Work out the finished part from the listing and answer in its coordinate system (mm). A direction names the side the tool comes from. Coordinates: 2 decimals unless noted, no trailing zeros. Write each loop counter-clockwise with the first axis right and the second up, starting at its lowest first coordinate (ties: lowest second). Pieces come first, ordered by that corner, then holes. Notation, with made-up numbers: (-30.75, 23) - (11.25, 23) arc R31 cw to (11.25, 53) - close; hole circle Ø6 at (87, 39.25). An arc over 180 degrees is marked (long way). Use a Markdown table: item, result. Add a question column.
(1) The part is cut by section A-A, the plane x = 0. Give the vertices of the cut face in (y, z).
(2) The part is cut by section D-D, the plane y = 7.75. Give the vertices of the cut face in (x, z) (3 decimals).
(3) A tool of negligible diameter and unlimited length cuts with its end or side. For faces 4 (the face through (0, 4, -4.45)), 5 (the face through (-2.961, 8.172, -1.915)), from which of +Z, -Z, +X, -X, +Y, -Y can it reach the whole face along a straight path? Write none if from no direction.
(4) Given pin 1 Ø5.5 at (x, y) = (0, 0) entering from -Z, flat-ended and moving along its own axis, determine where the tip first touches the part or whether it passes through.
(5) For a pull along Y with two mould halves and no side action, classify faces 1 (the face through (0, 10, 0)), 2 (the face through (2.5, 7.8, 0.55)), 3 (the face through (0, 4, 4.45)) as released by +Y, released by -Y, zero draft, split by the parting line, or undercut.
(6) The part is cut by section C-C, the plane z = 1.25. Give the vertices of the cut face in (x, y).
(7) Find the intervals of material crossed by line 1 (Y direction, x = 0, z = -2.8); line 2 (Y direction, x = 2.5, z = -2.3) (3 decimals); line 3 (X direction, y = 8, z = -3.5), in increasing order. Write a range as from..to.
(8) The part is cut by section B-B, the plane z = -3.25. Give the vertices of the cut face in (x, y) (3 decimals), then the cut area to 3 significant figures.
from build123d import *

# Parameters (mm, degrees)
SKETCH1_R                     = 3.05
BOSS_EXTRUDE1_DEPTH           = 4.45
BOSS_EXTRUDE1_DEPTH_BACK      = 4.45
TAP_DRILL_FOR_M1_6_TAP1_D     = 1.25
TAP_DRILL_FOR_M1_6_TAP1_DEPTH = 5
FILLET1_R                     = 1


with BuildPart() as part:
    # Sketch1 → Boss-Extrude1 (new body, two sides)
    with BuildSketch(Plane.XY) as boss_extrude1_sk:
        with BuildLine():
            Line((-5.4, 0), (-5.644394736, 10))
            Line((-5.644394736, 10), (5.644394736, 10))
            Line((5.644394736, 10), (5.4, 0))
            ThreePointArc((5.4, 0), (0, -5.4), (-5.4, 0))
        make_face()
        Circle(SKETCH1_R, mode=Mode.SUBTRACT)
    extrude(amount=BOSS_EXTRUDE1_DEPTH)
    extrude(boss_extrude1_sk.sketch, amount=-BOSS_EXTRUDE1_DEPTH_BACK)

    # Tap Drill for M1.6 Tap1
    with Locations(Plane(origin=(0, 0, -4.45), x_dir=(-1, 0, 0), z_dir=(0, 0, -1))):
        with Locations((-2.5, 7.75), (2.5, 7.75)):
            Hole(TAP_DRILL_FOR_M1_6_TAP1_D / 2, depth=TAP_DRILL_FOR_M1_6_TAP1_DEPTH)

    # Fillet1
    fillet1_edges = [part.edges().sort_by_distance(p)[0] for p in [
        (-5.644394736, 10, 0),
        (5.644394736, 10, 0),
    ]]
    fillet(fillet1_edges, radius=FILLET1_R)


solid = part.part
Model answer:
| question | item | result |
|---|---|---|
| 1 | outline | (-5.4, -4.45) - (-3.05, -4.45) - (-3.05, 4.45) - (-5.4, 4.45) - close; (3.05, -4.45) - (10, -4.45) - (10, 4.45) - (3.05, 4.45) - close |
| 2 | outline | (-5.589, -4.45) - (-3.125, -4.45) - (-3.125, 0.55) - (-1.875, 0.55) - (-1.875, -4.45) - (1.875, -4.45) - (1.875, 0.55) - (3.125, 0.55) - (3.125, -4.45) - (5.589, -4.45) - (5.589, 4.45) - (-5.589, 4.45) - close |
| 3 | face 4 | -Z, +X, -X, +Y, -Y |
| 3 | face 5 | -Z |
| 4 | pin 1 | through |
| 5 | face 1 | released by +Y |
| 5 | face 2 | undercut |
| 5 | face 3 | zero draft |
| 6 | outline | (-5.62, 8.98) - (-5.4, 0) arc R5.4 ccw to (5.4, 0) - (5.62, 8.98) arc R1 ccw to (4.62, 10) - (-4.62, 10) arc R1 ccw to start; hole circle Ø6.1 at (0, 0) |
| 7 | line 1 | -5.4..-3.05, 3.05..10 |
| 7 | line 2 | -4.786..-1.747, 1.747..7.125, 8.375..10 |
| 7 | line 3 | -5.6..-3.07, -1.93..1.93, 3.07..5.6 |
| 8 | outline | (-5.619, 8.976) - (-5.4, 0) arc R5.4 ccw to (5.4, 0) - (5.619, 8.976) arc R1 ccw to (4.62, 10) - (-4.62, 10) arc R1 ccw to start; hole circle Ø1.25 at (-2.5, 7.75); hole circle Ø6.1 at (0, 0); hole circle Ø1.25 at (2.5, 7.75) |
| 8 | area | 124 mm^2 |
